from build123d import *

# Parameters (mm, degrees)
BOSS_EXTRUDE1_DEPTH = 50
SKETCH2_R           = 5
CUT_EXTRUDE1_DEPTH  = 6


with BuildPart() as part:
    # Sketch1 → Boss-Extrude1 (new body)
    with BuildSketch(Plane.XY):
        with BuildLine():
            Line((-50, 15), (-25, 15))
            Line((-25, 15), (-25, 0))
            ThreePointArc((-25, 0), (0, -25), (25, 0))
            Line((25, 0), (25, 15))
            Line((25, 15), (50, 15))
            Line((50, 15), (50, 10))
            Line((50, 10), (30, 10))
            Line((30, 10), (30, 0))
            ThreePointArc((30, 0), (0, -30), (-30, 0))
            Line((-30, 0), (-30, 10))
            Line((-30, 10), (-50, 10))
            Line((-50, 10), (-50, 15))
        make_face()
    extrude(amount=BOSS_EXTRUDE1_DEPTH)

    # Sketch2 → Cut-Extrude1 (cut, through all)
    with BuildSketch(Plane.XZ.offset(-10)):
        with Locations((40, 37.5)):
            Circle(SKETCH2_R)
        with Locations((40, 12.5)):
            Circle(SKETCH2_R)
        with Locations((-40, 12.5)):
            Circle(SKETCH2_R)
        with Locations((-40, 37.5)):
            Circle(SKETCH2_R)
    extrude(amount=-CUT_EXTRUDE1_DEPTH, mode=Mode.SUBTRACT)


solid = part.part
Geometry check sheet. Reference: the model listing, model coordinates, mm. A direction names the side the tool comes from. Round coordinates to 2 decimals unless told otherwise and drop trailing zeros. Loops run counter-clockwise (first coordinate to the right, second up) from the corner with the lowest first, then second, coordinate; pieces in that order, holes last. Notation, with made-up numbers: (23, 29.25) - (31, 29.25) arc R16 ccw to (31, 60.25) - close; hole circle Ø5 at (33.5, 46.25). An arc over 180 degrees is marked (long way). Answer as CSV lines item,"result".
(1) Material ranges on line 1 along X through (y, z) = (5, 3); line 2 along Z through (x, y) = (40, 12.25); line 3 along X through (y, z) = (12, 37), recorded low to high.
Output values:
line 1,"x = -30 to -25, 25 to 30"
line 2,"z = 0 to 7.5, 17.5 to 32.5, 42.5 to 50"
line 3,"x = -50 to -44.97, -35.03 to -25, 25 to 35.03, 44.97 to 50"
(2) Cross-section at B-B, the plane x = -40. Enter the section's corners in (y, z), and give its area (3 significant figures).
Output values:
outline,"(10, 0) - (15, 0) - (15, 7.5) - (10, 7.5) - close; (10, 17.5) - (15, 17.5) - (15, 32.5) - (10, 32.5) - close; (10, 42.5) - (15, 42.5) - (15, 50) - (10, 50) - close"
area,"150 mm²"
(3) Cross-section at C-C, the plane z = 37.5. Enter the section's corners in (x, y).
Output values:
outline,"(-50, 10) - (-45, 10) - (-45, 15) - (-50, 15) - close; (-35, 10) - (-30, 10) - (-30, 0) arc R30 ccw to (30, 0) - (30, 10) - (35, 10) - (35, 15) - (25, 15) - (25, 0) arc R25 cw to (-25, 0) - (-25, 15) - (-35, 15) - close; (45, 10) - (50, 10) - (50, 15) - (45, 15) - close"
(4) Release check for a two-part mould opening along Z. For faces 4 (the face through (35.005, 12.465, 12.72)), 5 (the face through (-40, 10, 25)), 6 (the face through (-44.995, 12.465, 12.72)), 7 (the face through (8, -24, 0)) record: released by +Z, released by -Z, zero draft, split by the parting line, or undercut.
Output values:
face 4,"undercut"
face 5,"zero draft"
face 6,"undercut"
face 7,"released by -Z"
(5) Cross-section at D-D, the plane z = 19.5. Enter the section's corners in (x, y).
Output values:
outline,"(-50, 10) - (-30, 10) - (-30, 0) arc R30 ccw to (30, 0) - (30, 10) - (50, 10) - (50, 15) - (25, 15) - (25, 0) arc R25 cw to (-25, 0) - (-25, 15) - (-50, 15) - close"
(6) Set-up check for faces 1 (the face through (-30, 5, 25)), 2 (the face through (-25, 8, 25)), 3 (the face through (40, 10, 25)): record each of +Z, -Z, +X, -X, +Y, -Y from which the full face is reachable in a straight line by a thin tool's end or side.
Output values:
face 1,"+Z, -Z, -X, -Y"
face 2,"+Z, -Z, +Y"
face 3,"+Z, -Z, +X, -Y"
(7) Cross-section at A-A, the plane y = 8. Enter the section's corners in (x, z).
Output values:
outline,"(-30, 0) - (-25, 0) - (-25, 50) - (-30, 50) - close; (25, 0) - (30, 0) - (30, 50) - (25, 50) - close"
(8) Depth check by flat-ended pin: pin 1 Ø6 at (x, z) = (-40, 12.5) entering from +Y; pin 2 Ø7.5 at (y, z) = (5.5, 16) entering from -X; pin 3 Ø3 at (x, z) = (-36, 16) entering from -Y; pin 4 Ø1 at (x, z) = (-7.5, 14) entering from +Y. Enter the tip coordinate at first touch or a pass-through.
Output values:
pin 1,"passes through"
pin 2,"stops at x = -30"
pin 3,"stops at y = 10"
pin 4,"stops at y = -23.69"
